Here's how the part is built. I have some questions about the finished solid (model axes, mm). Round coordinates to 2 decimals unless told otherwise and drop trailing zeros. Loops run counter-clockwise (first coordinate to the right, second up) from the corner with the lowest first, then second, coordinate; pieces in that order, holes last. Notation, with made-up numbers: (32.25, 16.25) - (53.25, 16.25) arc R27 cw to (53.25, 39.25) - close; hole circle Ø10 at (29, -5.5). An arc over 180 degrees is marked (long way). Answer as a JSON object with one key per item and string values. Group by question number.
1) If I drill on line 1 along X through (y, z) = (7.75, -10); line 2 along Z through (x, y) = (290, 14.5), over which ranges is the centre line in solid material (lowest first)? Write a range as [from, to].
2) Will these pins go through, and if not, where does the flat tip stop? P1, Ø5, axis at x = 10, z = -190, coming from the -Y side; P2, Ø10, axis at x = 241.5, y = 15, coming from the +Z side.
3) I want a section at A-A, the plane z = -190. Please give me the cut outline in (x, y).
4) I want a section at B-B, the plane x = 10. Please give me the cut outline in (y, z).
from build123d import *

# Parameters (mm, degrees)
SKETCH1_W           = 300
SKETCH1_H           = 200
BOSS_EXTRUDE2_DEPTH = 20
SKETCH8_R           = 3
CUT_EXTRUDE14_DEPTH = 20
SKETCH10_R          = 3
CUT_EXTRUDE16_DEPTH = 20
SKETCH11_R          = 3
CUT_EXTRUDE17_DEPTH = 20


with BuildPart() as part:
    # Sketch1 → Boss-Extrude2 (new body)
    with BuildSketch(Plane(origin=(0, 0, 0), x_dir=(1, 0, 0), z_dir=(0, 1, 0))):
        with Locations((150, 100)):
            Rectangle(SKETCH1_W, SKETCH1_H)
    extrude(amount=BOSS_EXTRUDE2_DEPTH)

    # Sketch8 → Cut-Extrude14 (cut)
    with BuildSketch(Plane(origin=(0, 20, 0), x_dir=(1, 0, 0), z_dir=(0, 1, 0))):
        with Locations(Location((10, 190, 0), (0, 0, 270))):
            Circle(SKETCH8_R)
    extrude(amount=-CUT_EXTRUDE14_DEPTH, mode=Mode.SUBTRACT)

    # Sketch10 → Cut-Extrude16 (cut)
    with BuildSketch(Plane(origin=(0, 20, 0), x_dir=(1, 0, 0), z_dir=(0, 1, 0))):
        with Locations(Location((10, 10, 0), (0, 0, 270))):
            Circle(SKETCH10_R)
    extrude(amount=-CUT_EXTRUDE16_DEPTH, mode=Mode.SUBTRACT)

    # Sketch11 → Cut-Extrude17 (cut)
    with BuildSketch(Plane(origin=(0, 20, 0), x_dir=(1, 0, 0), z_dir=(0, 1, 0))):
        with Locations(Location((290, 190, 0), (0, 0, 270))):
            Circle(SKETCH11_R)
        with Locations(Location((290, 10, 0), (0, 0, 270))):
            Circle(SKETCH11_R)
    extrude(amount=-CUT_EXTRUDE17_DEPTH, mode=Mode.SUBTRACT)


solid = part.part
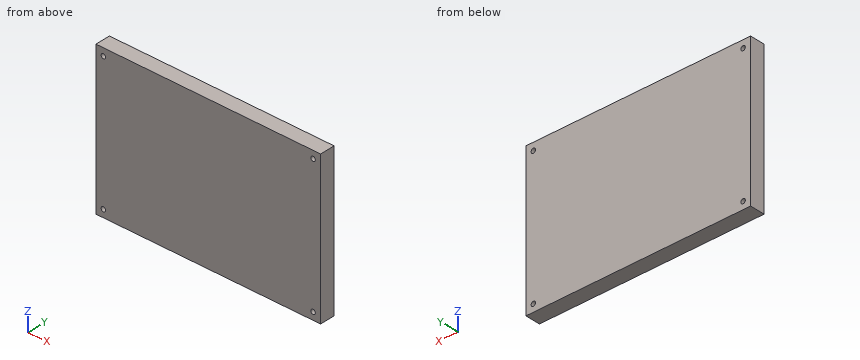
Outcome:
{
 "1": {"line 1": "[0, 7], [13, 287], [293, 300]", "line 2": "[-200, -193], [-187, -13], [-7, 0]"},
 "2": {"P1": "through", "P2": "z = 0"},
 "3": {"outline": "(0, 0) - (7, 0) - (7, 20) - (0, 20) - close; (13, 0) - (287, 0) - (287, 20) - (13, 20) - close; (293, 0) - (300, 0) - (300, 20) - (293, 20) - close"},
 "4": {"outline": "(0, -200) - (20, -200) - (20, -193) - (0, -193) - close; (0, -187) - (20, -187) - (20, -13) - (0, -13) - close; (0, -7) - (20, -7) - (20, 0) - (0, 0) - close"}
}
